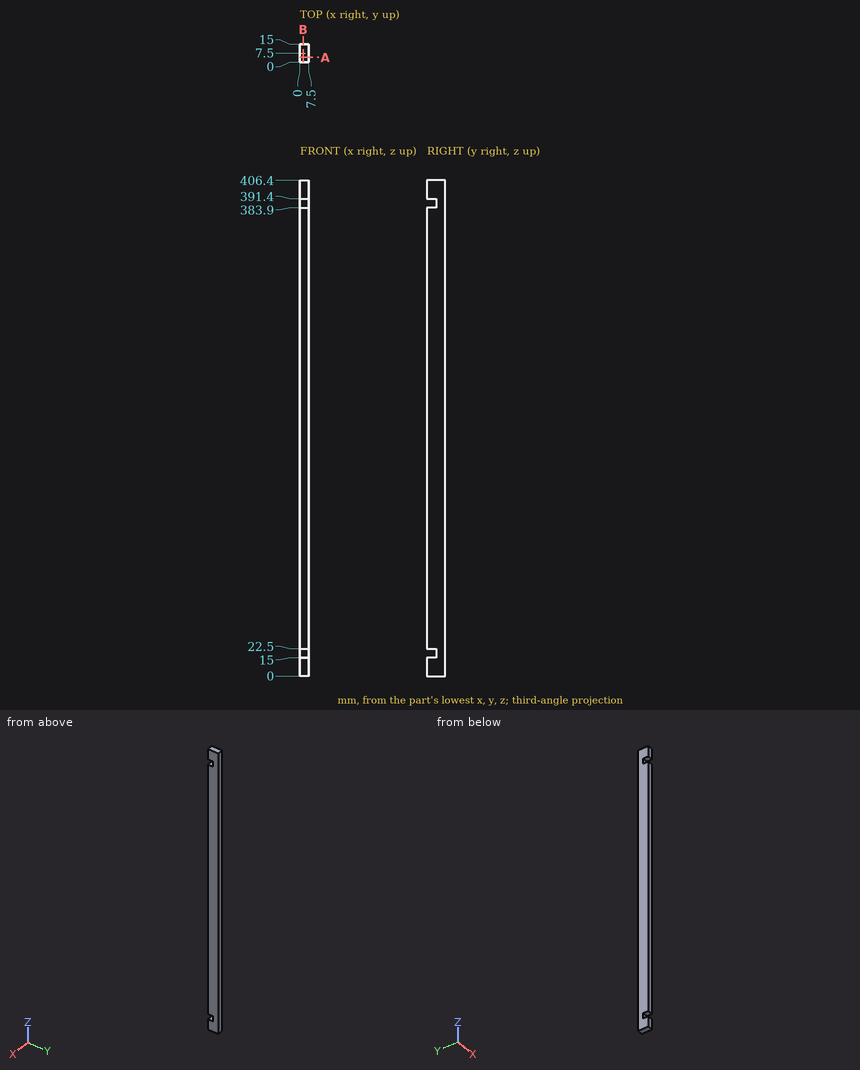
Job drawing, mm, ordinate dimensions from the low corner. One solid piece. Round coordinates to 2 decimals unless told otherwise and drop trailing zeros. Loops run counter-clockwise (first coordinate to the right, second up) from the corner with the lowest first, then second, coordinate; pieces in that order, holes last. Notation, with made-up numbers: M 60.5,42 L 68.5,42 A7 ccw 68.5,52 Z; hole C -36,37 d6. An arc over 180 degrees is marked long. Answer as CSV lines item,"result".
1. Wall check: probe 1 along Z at (x, y) = (1.75, 4.25). Give the ranges that are in metal, low to high. Write a range as [from, to].
Resolved:
probe 1,"z = [0, 15], [22.5, 383.9], [391.4, 406.4]"
2. Cut at A-A on y = 4. Write the cut outline in (x, z).
Resolved:
outline,"M 0,0 L 7.5,0 L 7.5,15 L 0,15 Z; M 0,22.5 L 7.5,22.5 L 7.5,383.9 L 0,383.9 Z; M 0,391.4 L 7.5,391.4 L 7.5,406.4 L 0,406.4 Z"
3. Flat gauge pin, fed straight in: P1, Ø2, axis at x = 2, z = 389, coming from the -Y side. Where does the tip first touch, or does it go through?
Resolved:
P1,"stops at y = 7.5"
4. Cut at B-B on x = 2.75. Write the cut outline in (y, z), then the cut area to 3 significant figures.
Resolved:
outline,"M 0,0 L 15,0 L 15,406.4 L 0,406.4 L 0,391.4 L 7.5,391.4 L 7.5,383.9 L 0,383.9 L 0,22.5 L 7.5,22.5 L 7.5,15 L 0,15 Z"
area,"5,980 mm²"
